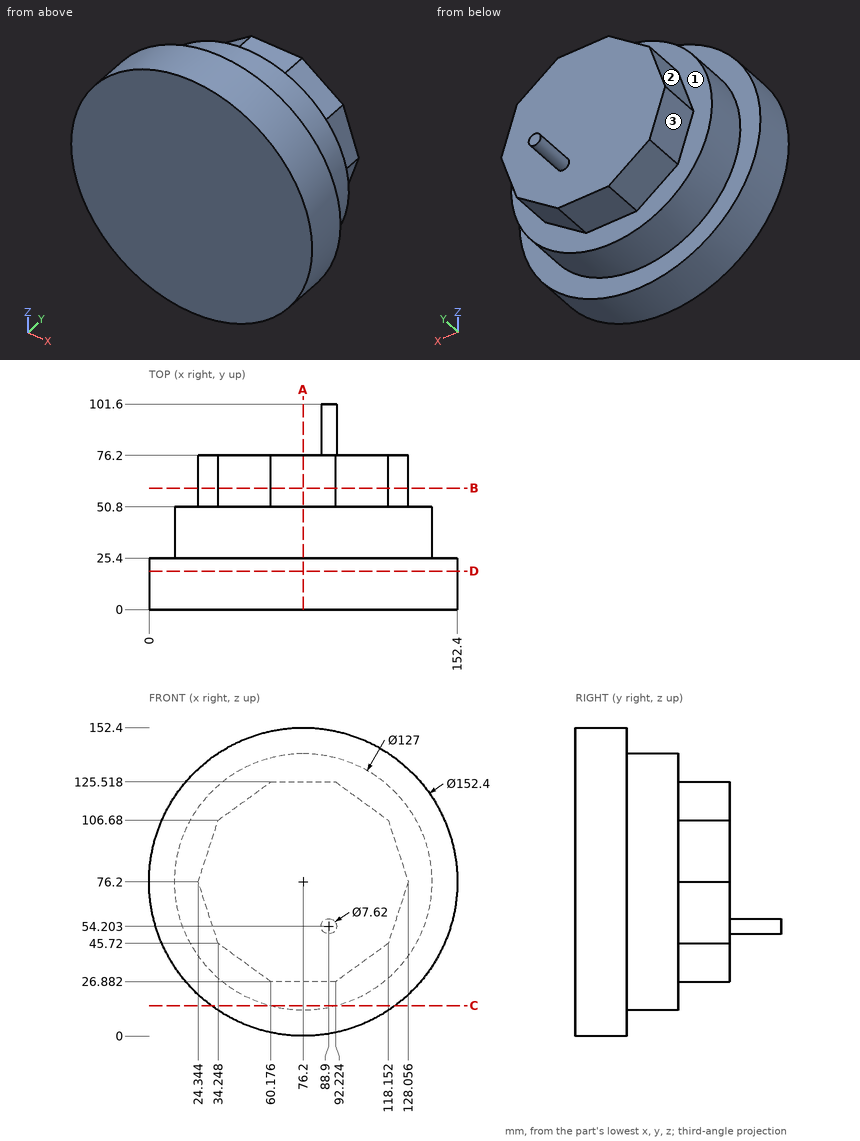
Input: dimensioned drawing with shaded views. Units: mm. Origin: part minimum x, y, z. A direction names the side the tool comes from. Give positions to 0.01 mm unless a question says otherwise; leave off trailing zeros. Write each loop counter-clockwise with the first axis right and the second up, starting at its lowest first coordinate (ties: lowest second). Pieces come first, ordered by that corner, then holes. Notation, with made-up numbers: M 87.25,-19.5 L 138.25,-19.5 A33 cw 138.25,18.5 Z; hole C 47,30.25 d10. An arc over 180 degrees is marked long. Return JSON: item names as keys, results as strings. Group by question number.
1) Cut plane A-A, the plane x = 76.2. Output: boundary loops of the cut face in (y, z), plus the area to 3 significant figures.
2) Cut plane B-B, the plane y = 60. Output: boundary loops of the cut face in (x, z), plus the area to 3 significant figures.
3) Pin query (flat end, axial travel): P1, Ø2, axis at y = 16.5, z = 62.5, coming from the +X side; P2, Ø2, axis at x = 75, z = 16, coming from the +Y side; P3, Ø20.5, axis at x = 76.5, y = 62, coming from the -Z side. Return the tip coordinate at first contact, or that it passes through.
4) Cut plane C-C, the plane z = 15. Output: boundary loops of the cut face in (x, y) (1 decimal).
5) Set-up query: the marked faces 1, 2 and 3. Return all of +Z, -Z, +X, -X, +Y, -Y with unobstructed straight access to the full face (end or side cutting, diameter ignored); none if empty.
6) Cut plane D-D, the plane y = 19. Output: boundary loops of the cut face in (x, z).
7) Material intervals for line 1 along Y through (x, z) = (28, 90); line 2 along Y through (x, z) = (55.5, 99); line 3 along X through (y, z) = (19, 78.5) (1 decimal), sorted ascending. Write a range as [from, to].
Recorded:
{
 "1": {"outline": "M 0,0 L 25.4,0 L 25.4,12.7 L 50.8,12.7 L 50.8,26.88 L 76.2,26.88 L 76.2,125.52 L 50.8,125.52 L 50.8,139.7 L 25.4,139.7 L 25.4,152.4 L 0,152.4 Z", "area": "9,600 mm²"},
 "2": {"outline": "M 24.34,76.2 L 34.25,45.72 L 60.18,26.88 L 92.22,26.88 L 118.15,45.72 L 128.06,76.2 L 118.15,106.68 L 92.22,125.52 L 60.18,125.52 L 34.25,106.68 Z", "area": "7,900 mm²"},
 "3": {"P1": "stops at x = 151.33", "P2": "stops at y = 50.8", "P3": "stops at z = 26.88"},
 "4": {"outline": "M 30.8,0 L 121.6,0 L 121.6,25.4 L 93.1,25.4 L 93.1,50.8 L 59.3,50.8 L 59.3,25.4 L 30.8,25.4 Z"},
 "5": {"face 1": "+Y", "face 2": "+Z, -X, +Y", "face 3": "-Z, -X, +Y"},
 "6": {"outline": "C 76.2,76.2 d152.4"},
 "7": {"line 1": "y = [0, 50.8]", "line 2": "y = [0, 76.2]", "line 3": "x = [0, 152.4]"}
}
